Design review of the part built by this model. Coordinates are the model's own, in mm. Face numbers are marked on the shaded views. A direction names the side the tool comes from. Give positions to 0.01 mm unless a question says otherwise; leave off trailing zeros. Order: outer loops, then holes, each group sorted by start corner. A loop starts at its lowest first (then second) coordinate and runs counter-clockwise, first axis right, second up. Notation, with made-up numbers: (-11.75, 23) -> (27.25, 23) arc R8 cw to (27.25, 29) -> close; hole circle Ø6 at (-0.75, -23). An arc over 180 degrees is marked (long way). Use a Markdown table: item, result. Add a question column.
```python
from build123d import *

# Parameters (mm, degrees)
F0_W      = 10.5
F0_H      = 10.5
F1_DEPTH  = 9
F2_R      = 3.0762
F3_DEPTH  = 5.135
F4_R      = 2.575
F5_DEPTH  = 25.4
F7_DEPTH  = 2
F8_R      = 1.675
F9_DEPTH  = 3
F10_SIZE  = 0.75
F11_R     = 0.625
F12_DEPTH = 4.5
F13_R     = 2.955
F14_DEPTH = 1.15


with BuildPart() as f1:
    # F0 (on Front) → F1 (new body)
    with BuildSketch(Plane.XZ):
        with Locations((5.25, 5.25)):
            Rectangle(F0_W, F0_H)
    extrude(amount=F1_DEPTH)

    # F2 (on face) → F3 (cut)
    with BuildSketch(Plane(origin=(0, 0, 0), x_dir=(0, -1, 0), z_dir=(-1, 0, 0))):
        with Locations((4.5, 4.5)):
            Circle(F2_R)
    extrude(amount=-F3_DEPTH, mode=Mode.SUBTRACT)

    # F4 (on face) → F5 (cut)
    with BuildSketch(Plane.YZ.offset(10.5)):
        with Locations((-4.5, 4.5)):
            Circle(F4_R)
    extrude(amount=-F5_DEPTH, mode=Mode.SUBTRACT)

    # F6 (on face) → F7 (cut)
    with BuildSketch(Plane.XY.offset(10.5)):
        with BuildLine():
            Line((2.85, -9), (10.5, -9))
            Line((10.5, -9), (10.5, -1.5))
            Line((10.5, -1.5), (3.35, -1.5))
            ThreePointArc((3.35, -1.5), (3.1, -1.75), (2.85, -1.5))
            Line((2.85, -1.5), (2.85, -9))
        make_face()
        with BuildLine():
            ThreePointArc((3.35, -1.5), (3.1, -1.25), (2.85, -1.5))
            Line((2.85, -1.5), (3.35, -1.5))
        make_face()
        with BuildLine():
            Line((3.35, -1.5), (2.85, -1.5))
            ThreePointArc((2.85, -1.5), (3.1, -1.75), (3.35, -1.5))
        make_face()
    extrude(amount=-F7_DEPTH, mode=Mode.SUBTRACT)

    # F8 (on face) → F9 (cut)
    with BuildSketch(Plane.XY.offset(8.5)):
        with Locations((7.075, -4.475)):
            Circle(F8_R)
    extrude(amount=-F9_DEPTH, mode=Mode.SUBTRACT)

    # F10
    f10_edges = [f1.edges().sort_by_distance(p)[0] for p in [
        (0, -4.5, 10.5),
        (5.25, 0, 0),
        (10.5, -0.75, 10.5),
    ]]
    chamfer(f10_edges, length=F10_SIZE)

    # F11 (on face) → F12 (cut)
    with BuildSketch(Plane(origin=(0, 0, 0), x_dir=(-1, 0, 0), z_dir=(0, 1, 0))):
        with Locations((-1.625, 8.875)):
            Circle(F11_R)
    extrude(amount=-F12_DEPTH, mode=Mode.SUBTRACT)

    # F13 (on face) → F14 (cut)
    with BuildSketch(Plane.YZ.offset(10.5)):
        with Locations((-4.5, 4.5)):
            Circle(F13_R)
    extrude(amount=-F14_DEPTH, mode=Mode.SUBTRACT)


solid = f1.part
```
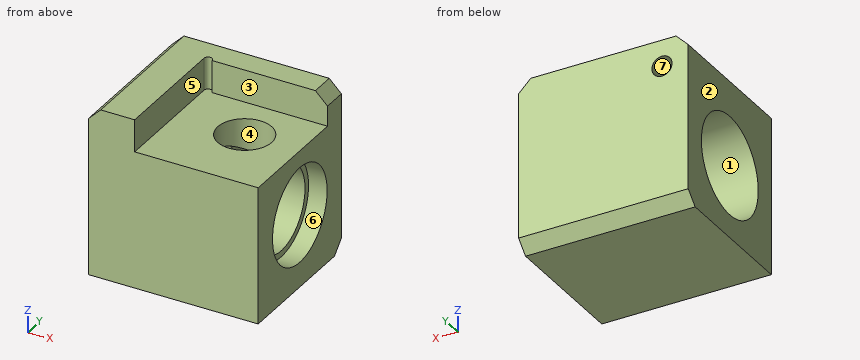
1) Add section B-B (z = 4.5). Give the boundary of the cut face in (x, y) (3 decimals).
2) Add section C-C (x = 3.1). Give the boundary of the cut face in (y, z).
3) Add section D-D (y = -5.25). Give the boundary of the cut face in (x, z) (3 decimals).
4) The part is to be moulded in two halves that separate along Y. For the marked faces 1, 2 and 3, say which applies: +Y half, -Y half, draft (parallel to the pull), parting line (faces both ways), or undercut.
5) For L1, parallel to Z at x = 2.6, y = -4.5; L2, parallel to Z at x = 3.95, y = -4.5; L3, parallel to X at y = -7, z = 3.75 (3 decimals), list the stretches that pass through material, from the lowest coordinate up. Write a range as [from, to].
6) Add section A-A (y = -3). Give the boundary of the cut face in (x, z) (3 decimals), then the cut area to 3 significant figures.
7) Machinability: for the marked faces 4, 5, 6 and 7, which of the approach directions +Z, -Z, +X, -X, +Y, -Y give a long, thin tool a straight path to every point of the face, cutting with its end or side? Answer none if there is none.
8) Insertion check: pin 1 (2 mm diameter, centred on y = -4.5, z = 10, fed in from +X); pin 2 (4.5 mm diameter, centred on y = -5, z = 4.5, fed in from +X); pin 3 (4 mm diameter, centred on x = 3.5, y = -5.5, fed in from +Z); pin 4 (4 mm diameter, centred on x = 7.075, y = -4.475, fed in from +Z). Each pin has a flat end and moves straight along its axis. Give the tip position at first contact, or say it passes through.
Worked answers:
| question | item | result |
|---|---|---|
| 1 | outline | (0, -9) -> (10.5, -9) -> (10.5, -7.455) -> (9.35, -7.455) -> (9.35, -7.075) -> (5.135, -7.075) -> (5.135, -7.576) -> (0, -7.576) -> close; (0, -1.424) -> (5.135, -1.424) -> (5.135, -1.925) -> (9.35, -1.925) -> (9.35, -1.545) -> (10.5, -1.545) -> (10.5, 0) -> (0, 0) -> close |
| 2 | outline | (-9, 0) -> (-0.75, 0) -> (0, 0.75) -> (0, 10.5) -> (-1.25, 10.5) -> (-1.25, 8.5) -> (-9, 8.5) -> close; hole circle Ø6.15 at (-4.5, 4.5) |
| 3 | outline | (0, 0) -> (10.5, 0) -> (10.5, 1.642) -> (9.35, 1.642) -> (9.35, 2.037) -> (5.135, 2.037) -> (5.135, 1.517) -> (0, 1.517) -> close; (0, 7.483) -> (5.135, 7.483) -> (5.135, 6.963) -> (5.59, 6.963) -> (5.59, 8.5) -> (2.85, 8.5) -> (2.85, 10.5) -> (0.75, 10.5) -> (0, 9.75) -> close; (8.56, 6.963) -> (9.35, 6.963) -> (9.35, 7.358) -> (10.5, 7.358) -> (10.5, 8.5) -> (8.56, 8.5) -> close |
| 4 | face 1 | undercut |
| 4 | face 2 | draft |
| 4 | face 3 | -Y half |
| 5 | L1 | [0, 1.42], [7.58, 10.5] |
| 5 | L2 | [0, 1.42], [7.58, 8.5] |
| 5 | L3 | [5.135, 9.35] |
| 6 | outline | (0, 0) -> (10.5, 0) -> (10.5, 1.954) -> (9.35, 1.954) -> (9.35, 2.407) -> (5.135, 2.407) -> (5.135, 1.814) -> (0, 1.814) -> close; (0, 7.186) -> (5.135, 7.186) -> (5.135, 6.593) -> (6.281, 6.593) -> (6.281, 8.5) -> (2.85, 8.5) -> (2.85, 10.5) -> (0.75, 10.5) -> (0, 9.75) -> close; (7.869, 6.593) -> (9.35, 6.593) -> (9.35, 7.046) -> (10.5, 7.046) -> (10.5, 8.5) -> (7.869, 8.5) -> close; hole circle Ø1.25 at (1.625, 8.875) |
| 6 | area | 39.3 mm^2 |
| 7 | face 4 | +Z |
| 7 | face 5 | +Z, +X, -Y |
| 7 | face 6 | +X |
| 7 | face 7 | +Y |
| 8 | pin 1 | x = 2.85 |
| 8 | pin 2 | x = 9.35 |
| 8 | pin 3 | z = 10.5 |
| 8 | pin 4 | z = 8.5 |
